Geometry check sheet. Reference: the model listing, model coordinates, mm. Face numbers are marked on the shaded views. Give positions to 0.01 mm unless a question says otherwise; leave off trailing zeros. Loops run counter-clockwise (first coordinate to the right, second up) from the corner with the lowest first, then second, coordinate; pieces in that order, holes last. Notation, with made-up numbers: (23.25, -6.5) -> (48.25, -6.5) arc R34 ccw to (48.25, 30.5) -> close; hole circle Ø7 at (85.5, 16). An arc over 180 degrees is marked (long way). Write item = value, one per line.
```python
from build123d import *

# Parameters (mm, degrees)
SKETCH1_W           = 45
SKETCH1_H           = 40
BOSS_EXTRUDE1_DEPTH = 28.91
SKETCH2_R           = 7.5
CUT_EXTRUDE1_DEPTH  = 189.461126468


with BuildPart() as part:
    # Sketch1 → Boss-Extrude1 (new body)
    with BuildSketch(Plane.XY):
        with Locations((159.384051224, 33.588569403)):
            Rectangle(SKETCH1_W, SKETCH1_H)
    extrude(amount=BOSS_EXTRUDE1_DEPTH)

    # Sketch2 → Cut-Extrude1 (cut, through all)
    with BuildSketch(Plane.XZ.offset(-13.588569403)):
        with Locations(Location((148.134051224, 16.25, 0), (0, 0, 270))):
            Circle(SKETCH2_R)
        with Locations(Location((170.634051224, 16.25, 0), (0, 0, 270))):
            Circle(SKETCH2_R)
    extrude(amount=-CUT_EXTRUDE1_DEPTH, mode=Mode.SUBTRACT)


solid = part.part
```
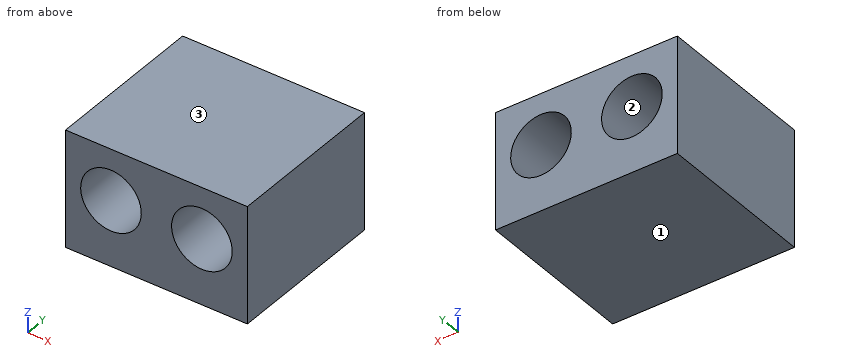
Item 1: Thickness scan on L1, parallel to X at y = 38, z = 16.25; L2, parallel to X at y = 17, z = 19.25; L3, parallel to Z at x = 167.5, y = 21. Record the ranges inside material, lowest first. Write a range as [from, to].
Answer:
L1 = [136.88, 140.63], [155.63, 163.13], [178.13, 181.88]
L2 = [136.88, 141.26], [155.01, 163.76], [177.51, 181.88]
L3 = [0, 9.44], [23.06, 28.91]
Item 2: Section check A-A, the plane x = 176. Record the cut outline in (y, z), plus the area to 3 significant figures.
Answer:
outline = (13.59, 0) -> (53.59, 0) -> (53.59, 11.01) -> (13.59, 11.01) -> close; (13.59, 21.49) -> (53.59, 21.49) -> (53.59, 28.91) -> (13.59, 28.91) -> close
area = 737 mm^2
Item 3: Section check D-D, the plane x = 154. Record the cut outline in (y, z), plus the area to 3 significant figures.
Answer:
outline = (13.59, 0) -> (53.59, 0) -> (53.59, 11.58) -> (13.59, 11.58) -> close; (13.59, 20.92) -> (53.59, 20.92) -> (53.59, 28.91) -> (13.59, 28.91) -> close
area = 783 mm^2
Item 4: Section check B-B, the plane z = 16.25. Record the cut outline in (x, y).
Answer:
outline = (136.88, 13.59) -> (140.63, 13.59) -> (140.63, 53.59) -> (136.88, 53.59) -> close; (155.63, 13.59) -> (163.13, 13.59) -> (163.13, 53.59) -> (155.63, 53.59) -> close; (178.13, 13.59) -> (181.88, 13.59) -> (181.88, 53.59) -> (178.13, 53.59) -> close
Item 5: Draft check along Z on the marked faces 1, 2 and 3. Enter one of: +Z half, -Z half, draft (parallel to the pull), parting line (faces both ways), or undercut.
Answer:
face_1 = -Z half
face_2 = undercut
face_3 = +Z half
Item 6: Section check C-C, the plane y = 16. Record the cut outline in (x, z), plus the area to 3 significant figures.
Answer:
outline = (136.88, 0) -> (181.88, 0) -> (181.88, 28.91) -> (136.88, 28.91) -> close; hole circle Ø15 at (148.13, 16.25); hole circle Ø15 at (170.63, 16.25)
area = 948 mm^2
Item 7: Gauge pin test, flat end, axial feed: pin 1 (10 mm diameter, centred on x = 145.5, z = 14, fed in from -Y). Record the tip position at first contact, or that the pin passes through.
Answer:
pin_1 = 13.59
